from build123d import *

# Parameters (mm, degrees)
SKETCH3_R           = 2.1
SKETCH3_R_2         = 2.6
BOSS_EXTRUDE1_DEPTH = 3.175
FILLET1_R           = 8


with BuildPart() as part:
    # Sketch3 → Boss-Extrude1 (new body)
    with BuildSketch(Plane(origin=(0, 0, 0), x_dir=(1, 0, 0), z_dir=(0, 1, 0))):
        Polygon((-35, -45), (35, -45), (35, -84.175), (77.25, -84.175), (77.25, -104.175), (57.25, -104.175), (57.25, -150.175), (-57.25, -150.175), (-57.25, -104.175), (-77.25, -104.175), (-77.25, -84.175), (-35, -84.175), align=None)
        with Locations((-25, -75)):
            Circle(SKETCH3_R, mode=Mode.SUBTRACT)
        with Locations((25, -75)):
            Circle(SKETCH3_R, mode=Mode.SUBTRACT)
        with Locations((-67.25, -94.175)):
            Circle(SKETCH3_R_2, mode=Mode.SUBTRACT)
        with Locations((67.25, -94.175)):
            Circle(SKETCH3_R_2, mode=Mode.SUBTRACT)
        with Locations((0, -134.175)):
            Circle(SKETCH3_R_2, mode=Mode.SUBTRACT)
    extrude(amount=BOSS_EXTRUDE1_DEPTH)

    # Fillet1
    fillet1_edges = [part.edges().sort_by_distance(p)[0] for p in [
        (35, 1.5875, 84.175),
        (77.25, 1.5875, 84.175),
        (77.25, 1.5875, 104.175),
        (57.25, 1.5875, 104.175),
        (57.25, 1.5875, 150.175),
        (-57.25, 1.5875, 150.175),
        (-57.25, 1.5875, 104.175),
        (-77.25, 1.5875, 104.175),
        (-77.25, 1.5875, 84.175),
        (-35, 1.5875, 84.175),
        (-35, 1.5875, 45),
        (35, 1.5875, 45),
    ]]
    fillet(fillet1_edges, radius=FILLET1_R)


solid = part.part
Could you check a few things on this model? Use its own coordinates, in mm. A direction names the side the tool comes from. Give positions to 0.01 mm unless a question says otherwise; leave off trailing zeros. Order: outer loops, then holes, each group sorted by start corner. A loop starts at its lowest first (then second) coordinate and runs counter-clockwise, first axis right, second up. Notation, with made-up numbers: (33, 5.25) -> (48, 5.25) arc R22 ccw to (48, 33.25) -> close; hole circle Ø11 at (71.25, 11). An arc over 180 degrees is marked (long way). Answer in a Markdown table with one row per item. Add a question column.
Item 1: Imagine slicing it at A-A (x = -25). List the corners of the cut face in (y, z) for me (3 decimals).
Item 2: Imagine slicing it at C-C (x = -67.25). List the corners of the cut face in (y, z) for me (3 decimals), and give its area (3 significant figures).
Item 3: Imagine slicing it at D-D (z = 118). List the corners of the cut face in (x, y) for me (3 decimals), and give its area (3 significant figures).
Item 4: For faces 1 (the flat face through (-67, 2, 104.175)), 2 (the flat face through (57.25, 2, 127)), 3 (the flat face through (-35, 2, 65)), which set-ups out of +Z, -Z, +X, -X, +Y, -Y let a thin tool reach every point of the face, with its end or its side?
Item 5: I'm going to push flat-ended pins straight in: P1, Ø3.5, axis at x = -25, z = 75, coming from the -Y side; P2, Ø1.6, axis at x = -67, y = 1, coming from the +Z side (3 decimals); P3, Ø1.6, axis at y = 1.5, z = 134, coming from the +X side; P4, Ø1.6, axis at y = 2, z = 66, coming from the -X side. Where does each tip first touch, or does it pass through?
Item 6: Please list where these lines run through material, in increasing order: probe 1 along X at (y, z) = (1.4, 75); probe 2 along Z at (x, y) = (25, 1.25) (3 decimals); probe 3 along Z at (x, y) = (0, 2) (3 decimals).
Item 7: Imagine slicing it at B-B (y = 2.3). Count the separate pieces of the cut face and the enclosed holes in it, and give its area (3 significant figures).
Result:
| question | item | result |
|---|---|---|
| 1 | outline | (0, 45) -> (3.175, 45) -> (3.175, 72.9) -> (0, 72.9) -> close; (0, 77.1) -> (3.175, 77.1) -> (3.175, 150.175) -> (0, 150.175) -> close |
| 2 | outline | (0, 84.175) -> (3.175, 84.175) -> (3.175, 91.575) -> (0, 91.575) -> close; (0, 96.775) -> (3.175, 96.775) -> (3.175, 104.175) -> (0, 104.175) -> close |
| 2 | area | 47.0 mm2 |
| 3 | outline | (-57.25, 0) -> (57.25, 0) -> (57.25, 3.175) -> (-57.25, 3.175) -> close |
| 3 | area | 364 mm2 |
| 4 | face 1 | +Z, -X, +Y, -Y |
| 4 | face 2 | +Z, +X, +Y, -Y |
| 4 | face 3 | -Z, -X, +Y, -Y |
| 5 | P1 | through |
| 5 | P2 | z = 104.175 |
| 5 | P3 | x = 57.25 |
| 5 | P4 | x = -35 |
| 6 | probe 1 | -35 to -27.1, -22.9 to 22.9, 27.1 to 35 |
| 6 | probe 2 | 45 to 72.9, 77.1 to 150.175 |
| 6 | probe 3 | 45 to 131.575, 136.775 to 150.175 |
| 7 | separate pieces | 1 |
| 7 | enclosed holes | 5 |
| 7 | area | 11,000 mm2 |
